```python
from build123d import *

# Parameters (mm, degrees)
SKIZZE1_R                       = 3.75
SKIZZE1_W                       = 33.75
SKIZZE1_H                       = 14
AUFSATZ_LINEAR_AUSTRAGEN1_DEPTH = 2
AUFSATZ_LINEAR_AUSTRAGEN2_DEPTH = 10
VERRUNDUNG1_R                   = 2
FASE2_SIZE                      = 1.5


with BuildPart() as part:
    # Skizze1 → Aufsatz-Linear austragen1 (new body)
    # profile 1 of 10: a face of its own
    with BuildSketch(Plane(origin=(0, 0, 0), x_dir=(1, 0, 0), z_dir=(0, 1, 0))):
        with BuildLine():
            Line((-15.125, 17.875), (15.125, 17.875))
            ThreePointArc((15.125, 17.875), (17.069543648, 17.069543648), (17.875, 15.125))
            Line((17.875, 15.125), (17.875, -15.125))
            ThreePointArc((17.875, -15.125), (17.069543648, -17.069543648), (15.125, -17.875))
            Line((15.125, -17.875), (-15.125, -17.875))
            ThreePointArc((-15.125, -17.875), (-17.069543648, -17.069543648), (-17.875, -15.125))
            Line((-17.875, -15.125), (-17.875, 15.125))
            ThreePointArc((-17.875, 15.125), (-17.069543648, 17.069543648), (-15.125, 17.875))
        make_face()
        with BuildLine():
            ThreePointArc((-15.125, 16.875), (-16.362436867, 16.362436867), (-16.875, 15.125))
            Line((-16.875, 15.125), (-16.875, -15.125))
            ThreePointArc((-16.875, -15.125), (-16.362436867, -16.362436867), (-15.125, -16.875))
            Line((-15.125, -16.875), (15.125, -16.875))
            ThreePointArc((15.125, -16.875), (16.362436867, -16.362436867), (16.875, -15.125))
            Line((16.875, -15.125), (16.875, 15.125))
            ThreePointArc((16.875, 15.125), (16.362436867, 16.362436867), (15.125, 16.875))
            Line((15.125, 16.875), (-15.125, 16.875))
        make_face(mode=Mode.SUBTRACT)
    # profile 2 of 10: a face of its own
    with BuildSketch(Plane(origin=(0, 0, 0), x_dir=(1, 0, 0), z_dir=(0, 1, 0))):
        with BuildLine():
            Line((16.875, -2.625), (-16.875, -2.625))
            Line((-16.875, -2.625), (-16.875, -15.125))
            ThreePointArc((-16.875, -15.125), (-16.362436867, -16.362436867), (-15.125, -16.875))
            Line((-15.125, -16.875), (15.125, -16.875))
            ThreePointArc((15.125, -16.875), (16.362436867, -16.362436867), (16.875, -15.125))
            Line((16.875, -15.125), (16.875, -2.625))
        make_face()
        with Locations(Location((0, -9.125, 0), (0, 0, 270))):
            Circle(SKIZZE1_R, mode=Mode.SUBTRACT)
    # profile 3 of 10: a face of its own
    with BuildSketch(Plane(origin=(0, 0, 0), x_dir=(1, 0, 0), z_dir=(0, 1, 0))):
        with Locations((0, 4.375)):
            Rectangle(SKIZZE1_W, SKIZZE1_H)
        with BuildLine():
            ThreePointArc((-12, 7.375), (-11.414213562, 8.789213562), (-10, 9.375))
            Line((-10, 9.375), (0, 9.375))
            Line((0, 9.375), (10, 9.375))
            ThreePointArc((10, 9.375), (11.414213562, 8.789213562), (12, 7.375))
            Line((12, 7.375), (12, 1.375))
            ThreePointArc((12, 1.375), (11.414213562, -0.039213562), (10, -0.625))
            Line((10, -0.625), (0, -0.625))
            Line((0, -0.625), (-10, -0.625))
            ThreePointArc((-10, -0.625), (-11.414213562, -0.039213562), (-12, 1.375))
            Line((-12, 1.375), (-12, 7.375))
        make_face(mode=Mode.SUBTRACT)
    # profile 4 of 10: a face of its own
    with BuildSketch(Plane(origin=(0, 0, 0), x_dir=(1, 0, 0), z_dir=(0, 1, 0))):
        Polygon((-12, 1.375), (0, -0.625), (12, 1.375), (12, 7.375), (0, 9.375), (-12, 7.375), align=None)
        Polygon((-10.5, 6.104309367), (-10.5, 2.645690633), (0, 0.895690633), (10.5, 2.645690633), (10.5, 6.104309367), (0, 7.854309367), align=None, mode=Mode.SUBTRACT)
    # profile 5 of 10: a face of its own
    with BuildSketch(Plane(origin=(0, 0, 0), x_dir=(1, 0, 0), z_dir=(0, 1, 0))):
        Polygon((-10.5, 6.104309367), (0, 7.854309367), (10.5, 6.104309367), (10.5, 2.645690633), (0, 0.895690633), (-10.5, 2.645690633), align=None)
    # profile 6 of 10: a face of its own
    with BuildSketch(Plane(origin=(0, 0, 0), x_dir=(1, 0, 0), z_dir=(0, 1, 0))):
        with BuildLine():
            Line((0, -0.625), (-12, 1.375))
            ThreePointArc((-12, 1.375), (-11.414213562, -0.039213562), (-10, -0.625))
            Line((-10, -0.625), (0, -0.625))
        make_face()
    # profile 7 of 10: a face of its own
    with BuildSketch(Plane(origin=(0, 0, 0), x_dir=(1, 0, 0), z_dir=(0, 1, 0))):
        with BuildLine():
            ThreePointArc((10, -0.625), (11.414213562, -0.039213562), (12, 1.375))
            Line((12, 1.375), (0, -0.625))
            Line((0, -0.625), (10, -0.625))
        make_face()
    # profile 8 of 10: a face of its own
    with BuildSketch(Plane(origin=(0, 0, 0), x_dir=(1, 0, 0), z_dir=(0, 1, 0))):
        with BuildLine():
            Line((10, 9.375), (0, 9.375))
            Line((0, 9.375), (12, 7.375))
            ThreePointArc((12, 7.375), (11.414213562, 8.789213562), (10, 9.375))
        make_face()
    # profile 9 of 10: a face of its own
    with BuildSketch(Plane(origin=(0, 0, 0), x_dir=(1, 0, 0), z_dir=(0, 1, 0))):
        with BuildLine():
            Line((0, 9.375), (-10, 9.375))
            ThreePointArc((-10, 9.375), (-11.414213562, 8.789213562), (-12, 7.375))
            Line((-12, 7.375), (0, 9.375))
        make_face()
    # profile 10 of 10: a face of its own
    with BuildSketch(Plane(origin=(0, 0, 0), x_dir=(1, 0, 0), z_dir=(0, 1, 0))):
        with BuildLine():
            Line((15.125, 16.875), (-15.125, 16.875))
            ThreePointArc((-15.125, 16.875), (-16.362436867, 16.362436867), (-16.875, 15.125))
            Line((-16.875, 15.125), (-16.875, 11.375))
            Line((-16.875, 11.375), (16.875, 11.375))
            Line((16.875, 11.375), (16.875, 15.125))
            ThreePointArc((16.875, 15.125), (16.362436867, 16.362436867), (15.125, 16.875))
        make_face()
    extrude(amount=AUFSATZ_LINEAR_AUSTRAGEN1_DEPTH)

    # Skizze1_6 → Aufsatz-Linear austragen2 (add)
    with BuildSketch(Plane(origin=(0, 0, 0), x_dir=(1, 0, 0), z_dir=(0, 1, 0))):
        Polygon((-12, 1.375), (0, -0.625), (12, 1.375), (12, 7.375), (0, 9.375), (-12, 7.375), align=None)
        Polygon((-10.5, 6.104309367), (-10.5, 2.645690633), (0, 0.895690633), (10.5, 2.645690633), (10.5, 6.104309367), (0, 7.854309367), align=None, mode=Mode.SUBTRACT)
    extrude(amount=-AUFSATZ_LINEAR_AUSTRAGEN2_DEPTH)

    # Verrundung1
    verrundung1_edges = [part.edges().sort_by_distance(p)[0] for p in [
        (0, -5, 0.625),
        (-12, -5, -1.375),
        (-12, -5, -7.375),
        (0, -5, -9.375),
        (12, -5, -7.375),
        (12, -5, -1.375),
    ]]
    fillet(verrundung1_edges, radius=VERRUNDUNG1_R)

    # Fase2
    fase2_edges = [part.edges().sort_by_distance(p)[0] for p in [
        (0, 2, 5.375),
    ]]
    chamfer(fase2_edges, length=FASE2_SIZE)


solid = part.part
```
Here's how the part is built. I have some questions about the finished solid (model axes, mm). A direction names the side the tool comes from. Coordinates: 2 decimals unless noted, no trailing zeros. Loops run counter-clockwise (first coordinate to the right, second up) from the corner with the lowest first, then second, coordinate; pieces in that order, holes last. Notation, with made-up numbers: M -25,-14.5 L 28,-14.5 A6 ccw 28,-7.5 Z; hole C -38,87 d6. An arc over 180 degrees is marked long. One line per item, written item: value.
1. Imagine slicing it at D-D (x = -8). List the corners of the cut face in (y, z) for me (3 decimals), and give its area (3 significant figures).
Geometry says:
outline: M -10,-8.042 L 0,-8.042 L 0,-17.875 L 2,-17.875 L 2,17.875 L 0,17.875 L 0,-0.708 L -10,-0.708 L -10,-2.229 L 0,-2.229 L 0,-6.521 L -10,-6.521 Z
area: 102 mm2
2. On a 3-axis mill with a long thin cutter (end or side, diameter ignored), from which of +Z, -Z, +X, -X, +Y, -Y can I reach the whole of each face in a straight line? I mean faces 4 (the cylindrical face through (-11.51, -5.07, -1.76)), 5 (the cylindrical face through (11.51, -5.07, -1.76)), 6 (the flat face through (5.399, -4.93, -8.475)), 7 (the flat face through (-5.18, -4.93, -6.99)). Say none if no direction works.
Geometry says:
face 4: +Z, -X, -Y
face 5: +Z, +X, -Y
face 6: -Z, +X, -Y
face 7: -Y
3. Imagine slicing it at A-A (y = -2). List the corners of the cut face in (x, z) for me.
Geometry says:
outline: M -12,-5.68 A2 ccw -10.33,-7.65 L -0.33,-9.32 A2 ccw 0.33,-9.32 L 10.33,-7.65 A2 ccw 12,-5.68 L 12,-3.07 A2 ccw 10.33,-1.1 L 0.33,0.57 A2 ccw -0.33,0.57 L -10.33,-1.1 A2 ccw -12,-3.07 Z; hole M -10.5,-6.1 L 0,-7.85 L 10.5,-6.1 L 10.5,-2.65 L 0,-0.9 L -10.5,-2.65 Z
4. Will these pins go through, and if not, where does the flat tip stop? pin 1 Ø1.3 at (y, z) = (-3, -5) entering from +X; pin 2 Ø6 at (x, z) = (-10, -11) entering from -Y; pin 3 Ø0.8 at (y, z) = (-3, -4.5) entering from -X; pin 4 Ø5 at (y, z) = (-7, 5.5) entering from -X.
Geometry says:
pin 1: stops at x = 12
pin 2: stops at y = 0
pin 3: stops at x = -12
pin 4: passes through
5. Please list where these lines run through material, in increasing order: probe 1 along X at (y, z) = (-1, -3); probe 2 along Z at (x, y) = (-6, -8) (3 decimals); probe 3 along Y at (x, z) = (3, -12.5).
Geometry says:
probe 1: x = -12 to -10.5, 10.5 to 12
probe 2: z = -8.375 to -6.854, -1.896 to -0.375
probe 3: y = 0 to 2
6. Thinking about a two-plate mould opening in Z: for faces 1 (the flat face through (10.5, -5, -4)), 2 (the flat face through (5.26, -4.93, -0.25)), 3 (the cylindrical face through (-17.09, 0.99, -17.05)), which applies, +Z half, -Z half, draft (parallel to the pull), parting line (faces both ways), or undercut?
Geometry says:
face 1: undercut
face 2: +Z half
face 3: -Z half
7. Imagine slicing it at C-C (z = -14.5). List the corners of the cut face in (x, y) for me (3 decimals), and give its area (3 significant figures).
Geometry says:
outline: M -17.875,0 L 17.875,0 L 17.875,2 L -17.875,2 Z
area: 71.5 mm2
8. Imagine slicing it at B-B (x = 11.5). List the corners of the cut face in (y, z) for me (3 decimals).
Geometry says:
outline: M -10,-7.004 L 0,-7.004 L 0,-17.875 L 2,-17.875 L 2,17.875 L 0,17.875 L 0,-1.746 L -10,-1.746 Z
